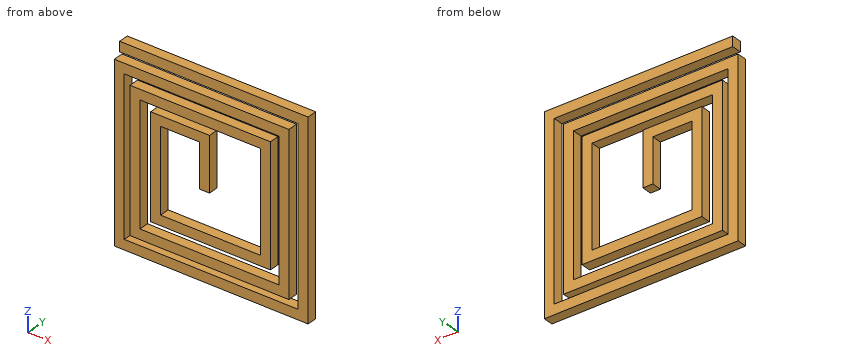
from build123d import *

# Parameters (mm, degrees)
SKETCH3_W = 7.046537748
SKETCH3_H = 7.046537748


with BuildPart() as part:
    # Sweep1: sweep along a path in Sketch2
    with BuildLine(Plane(origin=(0, 0, 0), x_dir=(1, 0, 0), z_dir=(0, 1, 0))) as sweep1_path:
        Line((-56.433512337, -33.614206506), (73.671403243, -33.614206506))
        Line((73.671403243, -33.614206506), (73.671403243, 96.490709074))
        Line((73.671403243, 96.490709074), (-56.731082257, 96.490709074))
        Line((-56.731082257, 96.490709074), (-56.731082257, -20.265698264))
        Line((-56.731082257, -20.265698264), (60.025325081, -20.265698264))
        Line((60.025325081, -20.265698264), (60.025325081, 85.412146694))
        Line((60.025325081, 85.412146694), (-45.652519877, 85.412146694))
        Line((-45.652519877, 85.412146694), (-45.652519877, -7.17127309))
        Line((-45.652519877, -7.17127309), (46.930899908, -7.17127309))
        Line((46.930899908, -7.17127309), (46.930899908, 70.729135959))
        Line((46.930899908, 70.729135959), (-30.969509142, 70.729135959))
        Line((-30.969509142, 70.729135959), (-30.969509142, 4.853856027))
        Line((-30.969509142, 4.853856027), (3.758736239, 4.853856027))
        Line((3.758736239, 4.853856027), (3.758736239, 39.582101408))
    # Sketch3 → Sweep1 (sweep)
    with BuildSketch(Plane(origin=(-56.433512337, 0, 0), x_dir=(0, 0, -1), z_dir=(1, 0, 0))):
        with Locations((-33.614206506, 0)):
            Rectangle(SKETCH3_W, SKETCH3_H)
    sweep(path=sweep1_path.line, transition=Transition.RIGHT)


solid = part.part
Can you work these out from the model? Positions are in its coordinate system, mm. Give positions to 0.01 mm unless a question says otherwise; leave off trailing zeros. Loops run counter-clockwise (first coordinate to the right, second up) from the corner with the lowest first, then second, coordinate; pieces in that order, holes last. Notation, with made-up numbers: (-9, 29) -> (44, 29) arc R28 cw to (44, 66) -> close; hole circle Ø6 at (-16.5, 85). An arc over 180 degrees is marked (long way). Return JSON: item names as keys, results as strings.
Q1. I want a section at C-C, the plane x = -19.5. List the corners of the cut face in (y, z) for me, then the cut area to 3 significant figures.
Checks:
{"outline": "(-3.52, -100.01) -> (3.52, -100.01) -> (3.52, -92.97) -> (-3.52, -92.97) -> close; (-3.52, -88.94) -> (3.52, -88.94) -> (3.52, -81.89) -> (-3.52, -81.89) -> close; (-3.52, -74.25) -> (3.52, -74.25) -> (3.52, -67.21) -> (-3.52, -67.21) -> close; (-3.52, -8.38) -> (3.52, -8.38) -> (3.52, -1.33) -> (-3.52, -1.33) -> close; (-3.52, 3.65) -> (3.52, 3.65) -> (3.52, 10.69) -> (-3.52, 10.69) -> close; (-3.52, 16.74) -> (3.52, 16.74) -> (3.52, 23.79) -> (-3.52, 23.79) -> close; (-3.52, 30.09) -> (3.52, 30.09) -> (3.52, 37.14) -> (-3.52, 37.14) -> close", "area": "348 mm2"}
Q2. I need wall thicknesses on probe 1 along X at (y, z) = (-1.75, -42); probe 2 along Z at (x, y) = (62.5, 2); probe 3 along Z at (x, y) = (-53, 1.5). Which ranges of each line are inside material? Lowest first, please.
Checks:
{"probe 1": "x = -60.25 to -53.21, -49.18 to -42.13, -34.49 to -27.45, 43.41 to 50.45, 56.5 to 63.55, 70.15 to 77.19", "probe 2": "z = -100.01 to -92.97, -88.94 to 23.79, 30.09 to 37.14", "probe 3": "z = -100.01 to -92.97, 16.74 to 23.79, 30.09 to 37.14"}
Q3. I want a section at B-B, the plane z = 20.5. List the corners of the cut face in (x, y) for me.
Checks:
{"outline": "(-60.25, -3.52) -> (63.55, -3.52) -> (63.55, 3.52) -> (-60.25, 3.52) -> close; (70.15, -3.52) -> (77.19, -3.52) -> (77.19, 3.52) -> (70.15, 3.52) -> close"}
Q4. I want a section at A-A, the plane x = 60. List the corners of the cut face in (y, z) for me.
Checks:
{"outline": "(-3.52, -100.01) -> (3.52, -100.01) -> (3.52, -92.97) -> (-3.52, -92.97) -> close; (-3.52, -88.94) -> (3.52, -88.94) -> (3.52, 23.79) -> (-3.52, 23.79) -> close; (-3.52, 30.09) -> (3.52, 30.09) -> (3.52, 37.14) -> (-3.52, 37.14) -> close"}
